The figure shows three views and two pictorial views of one solid part (mm, origin at its lowest corner). Answer the questions. Coordinates: 2 decimals unless noted, no trailing zeros. Loops run counter-clockwise (first coordinate to the right, second up) from the corner with the lowest first, then second, coordinate; pieces in that order, holes last. Notation, with made-up numbers: M -25.5,-13 L -1.5,-13 A16 ccw -1.5,-9 Z; hole C 55,64 d5. An arc over 180 degrees is marked long. Return JSON: item names as keys, results as strings. Group by question number.
1. The mould has two halves that part along Z. Classify the marked faces 1 and 2: pulls with the +Z half, pulls with the -Z half, needs draft (parallel to the pull), parting line crosses it, or undercut.
2. Given P1, Ø1.5, axis at x = 201, y = 643.5, coming from the -Z side; P2, Ø5, axis at y = 307.5, z = 235.5, coming from the +X side; P3, Ø8, axis at y = 543.5, z = 127, coming from the -X side, each flat-ended and moving along its own axis, determine where each tip first touches the part or whether it passes through.
3. Section B-B (z = 292) is taken. Write down the section's boundary in (x, y).
4. Section A-A (x = 133.5) is taken. Write down the section's boundary in (y, z) (1 decimal).
5. Straight lines are drawn through the part: L1, parallel to Z at x = 435, y = 398; L2, parallel to Z at x = 458.5, y = 450 (1 decimal); L3, parallel to X at y = 211.5, z = 68 (1 decimal). For each, find the intervals that lie inside material, in ascending order. Write a range as from..to.
6. Section D-D (x = 521.5) is taken. Write down the section's boundary in (y, z) (1 decimal).
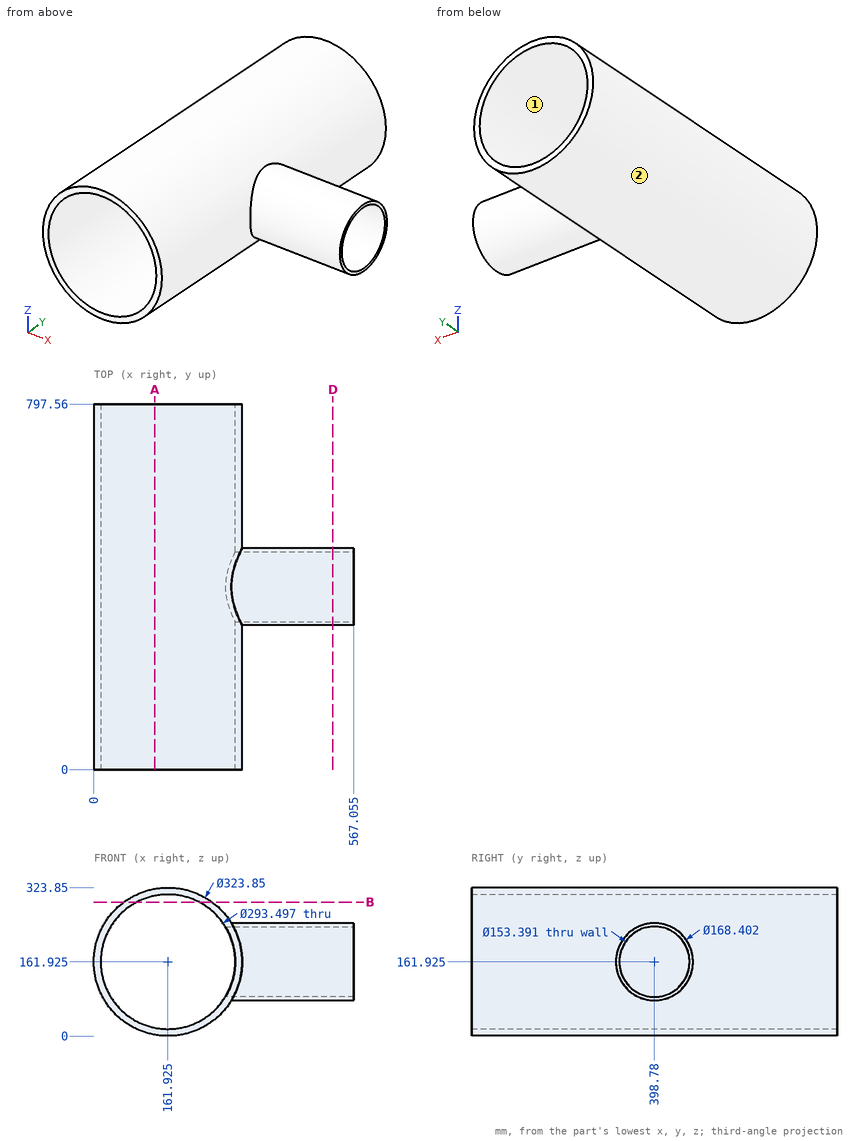
Worked out:
{
 "1": {"face 1": "undercut", "face 2": "parting line crosses it"},
 "2": {"P1": "z = 4.6", "P2": "x = 307.42", "P3": "x = 2.98"},
 "3": {"outline": "M 65.49,0 L 93.99,0 L 93.99,797.56 L 65.49,797.56 Z; M 229.86,0 L 258.36,0 L 258.36,797.56 L 229.86,797.56 Z"},
 "4": {"outline": "M 0,2.5 L 797.6,2.5 L 797.6,18 L 0,18 Z; M 0,305.9 L 797.6,305.9 L 797.6,321.3 L 0,321.3 Z"},
 "5": {"L1": "77.73..85.23, 238.62..246.12", "L2": "95.1..104.8, 219..228.8", "L3": "30..49.2, 274.7..293.8"},
 "6": {"outline": "C 398.8,161.9 d168.4; hole C 398.8,161.9 d153.4"}
}
